```python
from build123d import *

# Parameters (mm, degrees)
F1_DEPTH = 2.5
F2_W     = 10.3561575886
F2_H     = 0.5
F3_DEPTH = 3
F4_W     = 11.1018016556
F4_H     = 0.5
F5_DEPTH = 1
F6_DEPTH = 2.5
F7_W     = 3
F7_H     = 2.5
F8_DEPTH = 10


# Not quite as in the source:
# - after a boolean that leaves OpenCascade's solid faulty, fix() repairs it


with BuildPart() as f1:
    # F0 (on Front) → F1 (new body)
    with BuildSketch(Plane.XZ):
        with BuildLine():
            ThreePointArc((-1.5, 5.5509008278), (-3.4955328635, -4.5654955919), (5.75, 0))
            ThreePointArc((5.75, 0), (4.5654955919, 3.4955328635), (1.5, 5.5509008278))
            ThreePointArc((1.5, 5.5509008278), (0.7565779009, 5.7000078842), (0, 5.75))
            ThreePointArc((0, 5.75), (-0.7565779009, 5.7000078842), (-1.5, 5.5509008278))
        make_face()
    extrude(amount=F1_DEPTH)

    # F2 (on face) → F3 (join)
    with BuildSketch(Plane.XZ.offset(2.5)):
        with Locations((0, 2.25)):
            Rectangle(F2_W, F2_H)
        with Locations((0, -2.25)):
            Rectangle(F2_W, F2_H)
        with BuildLine():
            Line((5.1780787943, 2.5), (5.1780787943, 2))
            Line((5.1780787943, 2), (5.3909646632, 2))
            ThreePointArc((5.3909646632, 2), (5.2904319201, 2.2525163925), (5.1780787943, 2.5))
        make_face()
        with BuildLine():
            ThreePointArc((-5.1780787943, 2.5), (-5.2904319201, 2.2525163925), (-5.3909646632, 2))
            Line((-5.3909646632, 2), (-5.1780787943, 2))
            Line((-5.1780787943, 2), (-5.1780787943, 2.5))
        make_face()
        with BuildLine():
            Line((-5.1780787943, -2), (-5.3909646632, -2))
            ThreePointArc((-5.3909646632, -2), (-5.2904319201, -2.2525163925), (-5.1780787943, -2.5))
            Line((-5.1780787943, -2.5), (-5.1780787943, -2))
        make_face()
        with BuildLine():
            Line((5.3909646632, -2), (5.1780787943, -2))
            Line((5.1780787943, -2), (5.1780787943, -2.5))
            ThreePointArc((5.1780787943, -2.5), (5.2904319201, -2.2525163925), (5.3909646632, -2))
        make_face()
    extrude(amount=F3_DEPTH)

    # F4 (on face) → F5 (join)
    with BuildSketch(Plane(origin=(0, 0, 0), x_dir=(-1, 0, 0), z_dir=(0, 1, 0))):
        with Locations((0, 1.25)):
            Rectangle(F4_W, F4_H)
        with Locations((0, -1.25)):
            Rectangle(F4_W, F4_H)
        with BuildLine():
            Line((5.5509008278, 1.5), (5.5509008278, 1))
            Line((5.5509008278, 1), (5.6623758265, 1))
            ThreePointArc((5.6623758265, 1), (5.6122093093, 1.2512420505), (5.5509008278, 1.5))
        make_face()
        with BuildLine():
            Line((5.6623758265, -1), (5.5509008278, -1))
            Line((5.5509008278, -1), (5.5509008278, -1.5))
            ThreePointArc((5.5509008278, -1.5), (5.6122093093, -1.2512420505), (5.6623758265, -1))
        make_face()
        with BuildLine():
            Line((-5.5509008278, -1), (-5.6623758265, -1))
            ThreePointArc((-5.6623758265, -1), (-5.6122093093, -1.2512420505), (-5.5509008278, -1.5))
            Line((-5.5509008278, -1.5), (-5.5509008278, -1))
        make_face()
        with BuildLine():
            ThreePointArc((-5.5509008278, 1.5), (-5.6122093093, 1.2512420505), (-5.6623758265, 1))
            Line((-5.6623758265, 1), (-5.5509008278, 1))
            Line((-5.5509008278, 1), (-5.5509008278, 1.5))
        make_face()
    extrude(amount=F5_DEPTH)

    add(f1.part.fix(), mode=Mode.REPLACE)

    # F0 (on Front) → F6 (join)
    with BuildSketch(Plane.XZ):
        with BuildLine():
            ThreePointArc((0, 5.75), (0.7565779009, 5.7000078842), (1.5, 5.5509008278))
            Line((1.5, 5.5509008278), (1.5, 5.75))
            Line((1.5, 5.75), (0, 5.75))
        make_face()
        with BuildLine():
            Line((-1.5, 5.75), (-1.5, 5.5509008278))
            ThreePointArc((-1.5, 5.5509008278), (-0.7565779009, 5.7000078842), (0, 5.75))
            Line((0, 5.75), (-1.5, 5.75))
        make_face()
    extrude(amount=F6_DEPTH)

    # F7 (on face) → F8 (join)
    with BuildSketch(Plane.XY.offset(5.75)):
        with Locations((0, -1.25)):
            Rectangle(F7_W, F7_H)
    extrude(amount=F8_DEPTH)


solid = f1.part
```
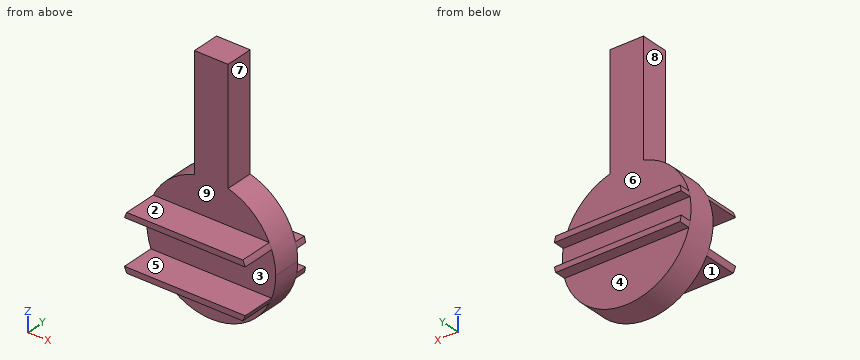
Can you work these out from the model? Positions are in its coordinate system, mm. Face numbers are marked on the shaded views. A direction names the side the tool comes from. Round coordinates to 2 decimals unless told otherwise and drop trailing zeros. Loops run counter-clockwise (first coordinate to the right, second up) from the corner with the lowest first, then second, coordinate; pieces in that order, holes last. Notation, with made-up numbers: M 74.25,25 L 121.25,25 A20 cw 121.25,59 Z; hole C 43,76 d4. An arc over 180 degrees is marked long. Answer in a Markdown table with one row per item.
1. Thinking about a two-plate mould opening in Z: for the marked faces 1, 2, 3 and 4, which applies, pulls with the +Z half, pulls with the -Z half, needs draft (parallel to the pull), parting line crosses it, or undercut?
Established:
| item | result |
|---|---|
| face 1 | pulls with the -Z half |
| face 2 | pulls with the +Z half |
| face 3 | undercut |
| face 4 | needs draft |
2. If we section it at A-A, the plane y = 0.5: Please give me the cut outline in (x, z), plus the area to 3 significant figures.
Established:
| item | result |
|---|---|
| outline | M -5.66,-1 A5.75 ccw -5.55,-1.5 L 5.55,-1.5 A5.75 ccw 5.66,-1 Z; M -5.66,1 L 5.66,1 A5.75 ccw 5.55,1.5 L -5.55,1.5 A5.75 ccw Z |
| area | 11.2 mm² |
3. I'm going to push flat-ended pins straight in: pin 1 Ø0.9 at (x, y) = (2.5, -4.5) entering from +Z; pin 2 Ø5.5 at (x, z) = (1.5, 10) entering from +Y; pin 3 Ø0.8 at (x, y) = (-2.5, 0.5) entering from +Z. Where does each tip first touch, or does it pass through?
Established:
| item | result |
|---|---|
| pin 1 | z = 2.5 |
| pin 2 | y = 0 |
| pin 3 | z = 1.5 |
4. If we section it at D-D, the plane x = -2.5: Please give me the cut outline in (y, z).
Established:
| item | result |
|---|---|
| outline | M -5.5,-2.5 L -2.5,-2.5 L -2.5,-5.18 L 0,-5.18 L 0,-1.5 L 1,-1.5 L 1,-1 L 0,-1 L 0,1 L 1,1 L 1,1.5 L 0,1.5 L 0,5.18 L -2.5,5.18 L -2.5,2.5 L -5.5,2.5 L -5.5,2 L -2.5,2 L -2.5,-2 L -5.5,-2 Z |
5. On a 3-axis mill with a long thin cutter (end or side, diameter ignored), from which of +Z, -Z, +X, -X, +Y, -Y can I reach the whole of each face in a straight line? I mean the marked faces 5, 6, 7, 8 and 9. Say none if no direction works.
Established:
| item | result |
|---|---|
| face 5 | +X, -X, -Y |
| face 6 | +Z, +X, -X, +Y |
| face 7 | +Z, +X, +Y, -Y |
| face 8 | +Z, -X, +Y, -Y |
| face 9 | +Z, +X, -X, -Y |
6. Please list where these lines run through material, in increasing order: line 1 (Z direction, x = 1.5, y = 0.25); line 2 (Z direction, x = 2.25, y = -5); line 3 (Y direction, x = -0.75, z = 12.5). Write a range as from..to.
Established:
| item | result |
|---|---|
| line 1 | -1.5..-1, 1..1.5 |
| line 2 | -2.5..-2, 2..2.5 |
| line 3 | -2.5..0 |
7. If we section it at B-B, the plane x = 0: Please give me the cut outline in (y, z).
Established:
| item | result |
|---|---|
| outline | M -5.5,-2.5 L -2.5,-2.5 L -2.5,-5.75 L 0,-5.75 L 0,-1.5 L 1,-1.5 L 1,-1 L 0,-1 L 0,1 L 1,1 L 1,1.5 L 0,1.5 L 0,15.75 L -2.5,15.75 L -2.5,2.5 L -5.5,2.5 L -5.5,2 L -2.5,2 L -2.5,-2 L -5.5,-2 Z |
8. If we section it at C-C, the plane y = -5: Please give me the cut outline in (x, z), plus the area to 3 significant figures.
Established:
| item | result |
|---|---|
| outline | M -5.39,-2 A5.75 ccw -5.18,-2.5 L 5.18,-2.5 A5.75 ccw 5.39,-2 Z; M -5.39,2 L 5.39,2 A5.75 ccw 5.18,2.5 L -5.18,2.5 A5.75 ccw Z |
| area | 10.6 mm² |
